from build123d import *

# Parameters (mm, degrees)
CROQUIS2_R                 = 9.525
CROQUIS2_R_2               = 8.5
SALIENTE_EXTRUIR1_DEPTH    = 50
CROQUIS3_R                 = 1.5875
CORTAR_EXTRUIR1_DEPTH      = 10.525
CORTAR_EXTRUIR1_DEPTH_BACK = 10.525


with BuildPart() as part:
    # Croquis2 → Saliente-Extruir1 (new body)
    with BuildSketch(Plane(origin=(0, 0, 0), x_dir=(1, 0, 0), z_dir=(0, 1, 0))):
        Circle(CROQUIS2_R)
        Circle(CROQUIS2_R_2, mode=Mode.SUBTRACT)
    extrude(amount=SALIENTE_EXTRUIR1_DEPTH)

    # Croquis3 → Cortar-Extruir1 (cut, two sides)
    with BuildSketch(Plane.XY) as cortar_extruir1_sk:
        with Locations((0, 42.0025)):
            Circle(CROQUIS3_R)
        with Locations((0, 8)):
            Circle(CROQUIS3_R)
    extrude(amount=CORTAR_EXTRUIR1_DEPTH, mode=Mode.SUBTRACT)
    extrude(cortar_extruir1_sk.sketch, amount=-CORTAR_EXTRUIR1_DEPTH_BACK, mode=Mode.SUBTRACT)


solid = part.part
Build history of the part. All positions in model axes, mm. Round coordinates to 2 decimals unless told otherwise and drop trailing zeros. Write each loop counter-clockwise with the first axis right and the second up, starting at its lowest first coordinate (ties: lowest second). Pieces come first, ordered by that corner, then holes. Notation, with made-up numbers: (62.5, 61.5) -> (83.5, 61.5) arc R13 ccw to (83.5, 82.5) -> close; hole circle Ø3 at (-19, -6). An arc over 180 degrees is marked (long way). Use one line per item in the form item = value.
Q1. Two-plate mould, pull along Y, no slides. Class faces 1 (the flat face through (-4, 50, -8)), 2 (the cylindrical face through (1.466, 41.394, -8.929)), 3 (the cylindrical face through (1.466, 7.392, -8.929)), 4 (the flat face through (-4, 0, -8)): released by +Y, released by -Y, zero draft, split by the parting line, or undercut.
Conclusion:
face_1 = released by +Y
face_2 = undercut
face_3 = undercut
face_4 = released by -Y
Q2. Band-saw the part on B-B, the plane x = 0. Write the cut outline in (y, z) (1 decimal), then the cut area to 3 significant figures.
Conclusion:
outline = (0, -9.5) -> (6.4, -9.5) -> (6.4, -8.5) -> (0, -8.5) -> close; (0, 8.5) -> (6.4, 8.5) -> (6.4, 9.5) -> (0, 9.5) -> close; (9.6, -9.5) -> (40.4, -9.5) -> (40.4, -8.5) -> (9.6, -8.5) -> close; (9.6, 8.5) -> (40.4, 8.5) -> (40.4, 9.5) -> (9.6, 9.5) -> close; (43.6, -9.5) -> (50, -9.5) -> (50, -8.5) -> (43.6, -8.5) -> close; (43.6, 8.5) -> (50, 8.5) -> (50, 9.5) -> (43.6, 9.5) -> close
area = 89.5 mm²
Q3. Drill centre lines: L1, parallel to Y at x = 0, z = 8.9 (1 decimal); L2, parallel to Z at x = 0, y = 36 (3 decimals). Where is each one in solid material? Low to high.
Conclusion:
L1 = 0 to 6.4, 9.6 to 40.4, 43.6 to 50
L2 = -9.525 to -8.5, 8.5 to 9.525
Q4. Band-saw the part on A-A, the plane z = 0. Write the cut outline in (x, y) (3 decimals).
Conclusion:
outline = (-9.525, 0) -> (-8.5, 0) -> (-8.5, 50) -> (-9.525, 50) -> close; (8.5, 0) -> (9.525, 0) -> (9.525, 50) -> (8.5, 50) -> close
Q5. Drop flat-ended pins along their axis: P1, Ø3, axis at x = -7, y = 21, coming from the -Z side; P2, Ø1, axis at y = 9.5, z = -6, coming from the +X side; P3, Ø3, axis at y = 8.5, z = -3.5, coming from the -X side; P4, Ø4, axis at x = 0.5, y = 32.5, coming from the -Z side (3 decimals). Give the stop position or say it passes through.
Conclusion:
P1 = -7.78
P2 = 7.78
P3 = -9.31
P4 = -9.525
Q6. Band-saw the part on D-D, the plane y = 45. Write the cut outline in (x, z) (3 decimals), then the cut area to 3 significant figures.
Conclusion:
outline = circle Ø19.05 at (0, 0); hole circle Ø17 at (0, 0)
area = 58.0 mm²
